from build123d import *

# Parameters (mm, degrees)
ESQUISSE1_R                     = 1.55
BOSS_EXTRU_2_DEPTH              = 6
R_P_TITION_LIN_AIRE1_COUNT      = 2
R_P_TITION_LIN_AIRE1_PITCH      = 7
R_P_TITION_LIN_AIRE1_COUNT_DIR2 = 5
R_P_TITION_LIN_AIRE1_PITCH_DIR2 = 7


with BuildPart() as part:
    # Esquisse1 → Boss.-Extru.2 (new body)
    with BuildSketch(Plane.XY):
        with BuildLine():
            Line((-0.25, 4.010434814), (-0.25, 2.989565186))
            ThreePointArc((-0.25, 2.989565186), (-2.121320344, 2.121320344), (-2.989565186, 0.25))
            Line((-2.989565186, 0.25), (-4.010434814, 0.25))
            ThreePointArc((-4.010434814, 0.25), (-4, 0), (-4.010434814, -0.25))
            Line((-4.010434814, -0.25), (-2.989565186, -0.25))
            ThreePointArc((-2.989565186, -0.25), (2.121320344, -2.121320344), (0.25, 2.989565186))
            Line((0.25, 2.989565186), (0.25, 4.010434814))
            ThreePointArc((0.25, 4.010434814), (0, 4), (-0.25, 4.010434814))
        make_face()
        Circle(ESQUISSE1_R, mode=Mode.SUBTRACT)
    boss_extru_2 = extrude(amount=BOSS_EXTRU_2_DEPTH)

    # Répétition linéaire1: Boss.-Extru.2 2 × 5
    with Locations(*[(j * R_P_TITION_LIN_AIRE1_PITCH_DIR2, -i * R_P_TITION_LIN_AIRE1_PITCH, 0) for i in range(R_P_TITION_LIN_AIRE1_COUNT) for j in range(R_P_TITION_LIN_AIRE1_COUNT_DIR2) if (i, j) != (0, 0)]):
        add(boss_extru_2)


solid = part.part
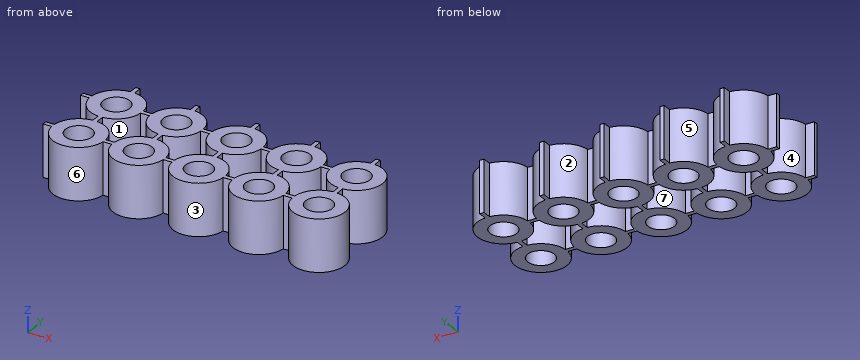
Verification items for the finished model (mm, model axes). Face numbers are marked on the shaded views. A direction names the side the tool comes from. Round coordinates to 2 decimals unless told otherwise and drop trailing zeros. Order: outer loops, then holes, each group sorted by start corner. A loop starts at its lowest first (then second) coordinate and runs counter-clockwise, first axis right, second up. Notation, with made-up numbers: (78.5, 84.5) -> (97.5, 84.5) arc R16 cw to (97.5, 110.5) -> close; hole circle Ø1 at (-26.5, 58). An arc over 180 degrees is marked (long way). Put each result on its own line as item: value.
1) Section check A-A (x = 22). Record the cut outline in (y, z), then the cut area to 3 significant figures.
Final values:
outline: (-9.83, 0) -> (-8.18, 0) -> (-8.18, 6) -> (-9.83, 6) -> close; (-5.82, 0) -> (-4.17, 0) -> (-4.17, 6) -> (-5.82, 6) -> close; (-2.83, 0) -> (-1.18, 0) -> (-1.18, 6) -> (-2.83, 6) -> close; (1.18, 0) -> (2.83, 0) -> (2.83, 6) -> (1.18, 6) -> close
area: 39.5 mm^2
2) Set-up check for the marked faces 1, 2, 3 and 4: record each of +Z, -Z, +X, -X, +Y, -Y from which the full face is reachable in a straight line by a thin tool's end or side.
Final values:
face 1: +Z, -Z
face 2: +Z, -Z, +Y
face 3: +Z, -Z, -Y
face 4: +Z, -Z, -X
3) Depth check by flat-ended pin: pin 1 (3 mm diameter, centred on x = 0, y = 0, fed in from -Z); pin 2 (0.8 mm diameter, centred on x = 10.5, z = 2, fed in from -Y); pin 3 (0.8 mm diameter, centred on x = 3.5, z = 2.5, fed in from +Y); pin 4 (1 mm diameter, centred on x = 26.5, z = 3.5, fed in from -Y). Enter the tip coordinate at first touch or a pass-through.
Final values:
pin 1: passes through
pin 2: stops at y = -7.25
pin 3: stops at y = 0.25
pin 4: stops at y = -9.83
4) Mould release check, pull along Y, two halves, no side actions. Record for the marked faces 5, 6 and 7: +Y half, -Y half, draft (parallel to the pull), parting line (faces both ways), or undercut.
Final values:
face 5: +Y half
face 6: -Y half
face 7: undercut
5) Material ranges on line 1 (X direction, y = -3.5, z = 2.95); line 2 (X direction, y = 2.5, z = 3.7); line 3 (Y direction, x = -1, z = 1.75), recorded low to high.
Final values:
line 1: x = -0.25 to 0.25, 6.75 to 7.25, 13.75 to 14.25, 20.75 to 21.25, 27.75 to 28.25
line 2: x = -1.66 to 1.66, 5.34 to 8.66, 12.34 to 15.66, 19.34 to 22.66, 26.34 to 29.66
line 3: y = -9.83 to -8.18, -5.82 to -4.17, -2.83 to -1.18, 1.18 to 2.83
6) Section check B-B (z = 2.9). Give the number of separate pieces and of enclosed holes in the cut face, then the cut area to 3 significant figures.
Final values:
separate pieces: 1
enclosed holes: 14
area: 217 mm^2
